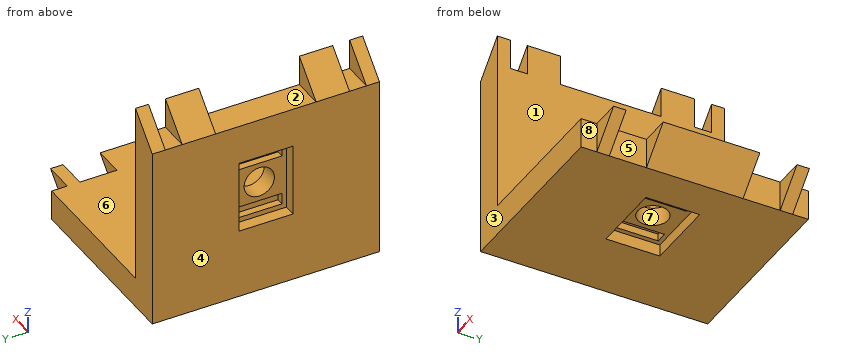
```python
from build123d import *

# Parameters (mm, degrees)
BOSS_EXTRUDE1_DEPTH      = 31.75
BOSS_EXTRUDE1_DEPTH_BACK = 6.35
BODY_MOVE_COPY1_ANGLE    = 90
SKETCH24_W               = 5.08
SKETCH24_H               = 2.84
SKETCH24_H_2             = 16.856
SKETCH24_H_3             = 2.839999908
CUT_EXTRUDE4_DEPTH       = 64.461888563
SKETCH26_W               = 5.08
SKETCH26_H               = 6.225000088
SKETCH26_H_2             = 2.629999912
CUT_EXTRUDE5_DEPTH       = 54.536186827
CHAMFER1_SIZE            = 5.08
CHAMFER2_SIZE            = 5.08
SKETCH29_W               = 12.0839992
SKETCH29_H               = 9.0359992
CUT_EXTRUDE6_DEPTH       = 2
SKETCH28_W               = 12.16937175
SKETCH28_H               = 9.099837858
CUT_EXTRUDE7_DEPTH       = 2
CUT_EXTRUDE8_REACH       = 66.997
SKETCH38_R               = 2.54
CUT_EXTRUDE10_REACH      = 57.348
SKETCH40_R               = 2.54
SKETCH41_W               = 1.905
SKETCH41_H               = 7.62
CUT_EXTRUDE11_DEPTH      = 1.2
SKETCH42_W               = 1.905
SKETCH42_H               = 7.62
CUT_EXTRUDE12_DEPTH      = 1.2


with BuildPart() as part:
    # Sketch1 → Boss-Extrude1 (new, two sides: drawn at the far end of the back side and taken through both)
    with BuildSketch(Plane(origin=(0, 0, 0), x_dir=(1, 0, 0), z_dir=(0, 1, 0)).offset(-BOSS_EXTRUDE1_DEPTH_BACK)):
        Polygon((0, 0), (30.48, 0), (30.48, -5.08), (-5.08, -5.08), (-5.08, 30.48), (0, 30.48), align=None)
    extrude(amount=BOSS_EXTRUDE1_DEPTH + BOSS_EXTRUDE1_DEPTH_BACK)


with BuildPart() as part_1:
    # Body-Move/Copy1: moved
    add(part.part.rotate(Axis((-5.08, 0, 5.08), (0, -1, 0)), BODY_MOVE_COPY1_ANGLE))


with BuildPart() as part_2:
    # Body-Move/Copy2: moved
    add(part_1.part.moved(Location((0, 0, -25.4))))


with BuildPart() as part_3:
    # Body-Move/Copy3: moved
    add(part_2.part.moved(Location((0, 0, -25.4))))

    # Sketch24 → Cut-Extrude4 (cut, through all)
    with BuildSketch(Plane(origin=(0, 0, 0), x_dir=(0, 0, -1), z_dir=(1, 0, 0))):
        with Locations((12.7, 28.15)):
            Rectangle(SKETCH24_W, SKETCH24_H)
        with Locations((12.7, 12.7)):
            Rectangle(SKETCH24_W, SKETCH24_H_2)
        with Locations((12.7, -2.75)):
            Rectangle(SKETCH24_W, SKETCH24_H_3)
    extrude(amount=-CUT_EXTRUDE4_DEPTH, mode=Mode.SUBTRACT)

    # Sketch26 → Cut-Extrude5 (cut, through all)
    with BuildSketch(Plane.XY.offset(-40.64)):
        with Locations((27.94, 23.9175)):
            Rectangle(SKETCH26_W, SKETCH26_H)
        with Locations((27.94, 30.435000044)):
            Rectangle(SKETCH26_W, SKETCH26_H_2)
        with Locations((27.94, 1.4825)):
            Rectangle(SKETCH26_W, SKETCH26_H)
        with Locations((27.94, -5.035000044)):
            Rectangle(SKETCH26_W, SKETCH26_H_2)
    extrude(amount=-CUT_EXTRUDE5_DEPTH, mode=Mode.SUBTRACT)

    # Chamfer1
    chamfer1_edges = [part_3.edges().sort_by_distance(p)[0] for p in [
        (-5.08, -5.259999977, -10.16),
        (-5.08, 1.470999977, -10.16),
        (-5.08, 23.929, -10.16),
        (-5.08, 30.66, -10.16),
    ]]
    chamfer(chamfer1_edges, length=CHAMFER1_SIZE - 0.0001)  # a hair under: the kernel refuses the full size

    # Chamfer2
    chamfer2_edges = [part_3.edges().sort_by_distance(p)[0] for p in [
        (30.48, -2.675000066, -45.72),
        (30.48, 12.7, -45.72),
        (30.48, 28.075000066, -45.72),
    ]]
    chamfer(chamfer2_edges, length=CHAMFER2_SIZE - 0.0001)  # a hair under: the kernel refuses the full size

    # Sketch29 → Cut-Extrude6 (cut)
    with BuildSketch(Plane(origin=(0, 0, -45.72), x_dir=(-1, 0, 0), z_dir=(0, 0, -1))):
        with Locations((-12.7, 12.7)):
            Rectangle(SKETCH29_W, SKETCH29_H)
    extrude(amount=-CUT_EXTRUDE6_DEPTH, mode=Mode.SUBTRACT)

    # Sketch28 → Cut-Extrude7 (cut)
    with BuildSketch(Plane.ZY.offset(5.08)):
        with Locations((-27.94, 12.682393608)):
            Rectangle(SKETCH28_W, SKETCH28_H)
    extrude(amount=-CUT_EXTRUDE7_DEPTH, mode=Mode.SUBTRACT)

    # Sketch38 → Cut-Extrude8 (cut, up to next)
    with BuildSketch(Plane.ZY.offset(3.08), mode=Mode.PRIVATE) as cut_extrude8_sk1:
        with Locations((-27.94, 12.7)):
            Circle(SKETCH38_R)
    cut_extrude8_tool1 = extrude(cut_extrude8_sk1.sketch, amount=-CUT_EXTRUDE8_REACH, mode=Mode.PRIVATE) & part_3.part
    add(cut_extrude8_tool1.solids().sort_by_distance((-3.08, 12.7, -27.94))[0], mode=Mode.SUBTRACT)

    # Sketch40 → Cut-Extrude10 (cut, up to next)
    with BuildSketch(Plane(origin=(0, 0, -43.72), x_dir=(-1, 0, 0), z_dir=(0, 0, -1)), mode=Mode.PRIVATE) as cut_extrude10_sk1:
        with Locations((-12.717733491, 12.7)):
            Circle(SKETCH40_R)
    cut_extrude10_tool1 = extrude(cut_extrude10_sk1.sketch, amount=-CUT_EXTRUDE10_REACH, mode=Mode.PRIVATE) & part_3.part
    add(cut_extrude10_tool1.solids().sort_by_distance((12.717733, 12.7, -43.72))[0], mode=Mode.SUBTRACT)

    # Sketch41 → Cut-Extrude11 (cut)
    with BuildSketch(Plane(origin=(0, 0, -43.72), x_dir=(-1, 0, 0), z_dir=(0, 0, -1))):
        with Locations((-8.400133455, 12.7)):
            Rectangle(SKETCH41_W, SKETCH41_H)
        with Locations((-16.999866545, 12.7)):
            Rectangle(SKETCH41_W, SKETCH41_H)
    extrude(amount=-CUT_EXTRUDE11_DEPTH, mode=Mode.SUBTRACT)

    # Sketch42 → Cut-Extrude12 (cut)
    with BuildSketch(Plane.ZY.offset(3.08)):
        with Locations((-23.640133455, 12.7)):
            Rectangle(SKETCH42_W, SKETCH42_H)
        with Locations((-32.239866545, 12.7)):
            Rectangle(SKETCH42_W, SKETCH42_H)
    extrude(amount=-CUT_EXTRUDE12_DEPTH, mode=Mode.SUBTRACT)


solid = part_3.part
```
The listing builds one solid part. Answer for the finished solid, in the listing's coordinates (mm). Face numbers are marked on the shaded views. A direction names the side the tool comes from. Coordinates: 2 decimals unless noted, no trailing zeros. Write each loop counter-clockwise with the first axis right and the second up, starting at its lowest first coordinate (ties: lowest second). Pieces come first, ordered by that corner, then holes. Notation, with made-up numbers: (-18, -15) - (35, -15) arc R24 cw to (35, -5) - close; hole circle Ø5 at (77, 35). An arc over 180 degrees is marked (long way). Return JSON: item names as keys, results as strings. Group by question number.
Q1. The part is cut by section C-C on x = 26.5. Write down the section's boundary in (y, z) (3 decimals), and give its area (3 significant figures).
Q2. Find the intervals of material crossed by line 1 along X through (y, z) = (-3, -25.5); line 2 along Z through (x, y) = (0.5, 30); line 3 along Y through (x, z) = (-1, -27), in increasing order. Write a range as [from, to].
Q3. Which of the six approach directions +Z, -Z, +X, -X, +Y, -Y give full straight-line access (tool end or side, diameter ignored) to the marked faces 1, 2, 3, 4 and 5?
Q4. The part is cut by section D-D on y = 12.7. State how many separate pieces and enclosed holes the cut face has, and give its area (3 significant figures).
Q5. For a pull along X with two mould halves and no side action, classify the marked faces 6, 7 and 8 as +X half, -X half, draft (parallel to the pull), parting line (faces both ways), or undercut.
Q6. The part is cut by section A-A on z = -27.94. Write down the section's boundary in (x, y).
Q7. Flat-ended cylindrical pins translate along their axes: pin 1 Ø1 at (y, z) = (14, -32.5) entering from -X; pin 2 Ø1.5 at (x, z) = (28, -43.5) entering from -Y; pin 3 Ø4.5 at (y, z) = (14.5, -29.5) entering from -X. Find the tip coordinate at first contact, or state that the pin passes through.
Evaluation:
{
 "1": {"outline": "(-3.72, -44.62) - (-1.63, -44.62) - (-1.63, -40.64) - (-3.72, -40.64) - close; (4.595, -44.62) - (20.805, -44.62) - (20.805, -40.64) - (4.595, -40.64) - close; (27.03, -44.62) - (29.12, -44.62) - (29.12, -40.64) - (27.03, -40.64) - close", "area": "81.2 mm2"},
 "2": {"line 1": "x = [-5.08, 0]", "line 2": "z = [-45.72, -40.64]", "line 3": "y = [-6.35, 10.34], [15.06, 31.75]"},
 "3": {"face 1": "+Z, +X, +Y, -Y", "face 2": "+Z, +X, -X", "face 3": "+Z, -Z, +X, -X, -Y", "face 4": "+Z, -Z, -X, +Y, -Y", "face 5": "+Z, -Z, +X"},
 "4": {"separate pieces": "3", "enclosed holes": "0", "area": "208 mm2"},
 "5": {"face 6": "draft", "face 7": "undercut", "face 8": "+X half"},
 "6": {"outline": "(-5.08, -6.35) - (0, -6.35) - (0, 10.16) - (-3.08, 10.16) - (-3.08, 8.13) - (-5.08, 8.13) - close; (-5.08, 17.23) - (-3.08, 17.23) - (-3.08, 15.24) - (0, 15.24) - (0, 31.75) - (-5.08, 31.75) - close"},
 "7": {"pin 1": "stops at x = -1.88", "pin 2": "stops at y = -3.72", "pin 3": "stops at x = -3.08"}
}
